from build123d import *

# Parameters (mm, degrees)
SKETCH2_R          = 4.7625
SKETCH3_R          = 1.7272
CUT_EXTRUDE1_DEPTH = 12.7


with BuildPart() as part:
    # Base-Sweep: sweep along a path in Sketch1
    with BuildLine(Plane(origin=(0, 0, 0), x_dir=(0, 0, -1), z_dir=(1, 0, 0))) as base_sweep_path:
        Line((0, 0), (0, 21.59))
        ThreePointArc((0, 21.59), (1.859871939, 26.080128061), (6.35, 27.94))
        Line((6.35, 27.94), (82.55, 27.94))
        ThreePointArc((82.55, 27.94), (87.040128061, 26.080128061), (88.9, 21.59))
        Line((88.9, 21.59), (88.9, 0))
    # Sketch2 → Base-Sweep (sweep)
    with BuildSketch(Plane(origin=(0, 0, 0), x_dir=(1, 0, 0), z_dir=(0, 1, 0))):
        Circle(SKETCH2_R)
    sweep(path=base_sweep_path.line)

    # Sketch3 → Cut-Extrude1 (cut)
    with BuildSketch(Plane.XZ):
        Circle(SKETCH3_R)
        with Locations((0, -88.9)):
            Circle(SKETCH3_R)
    extrude(amount=-CUT_EXTRUDE1_DEPTH, mode=Mode.SUBTRACT)


solid = part.part
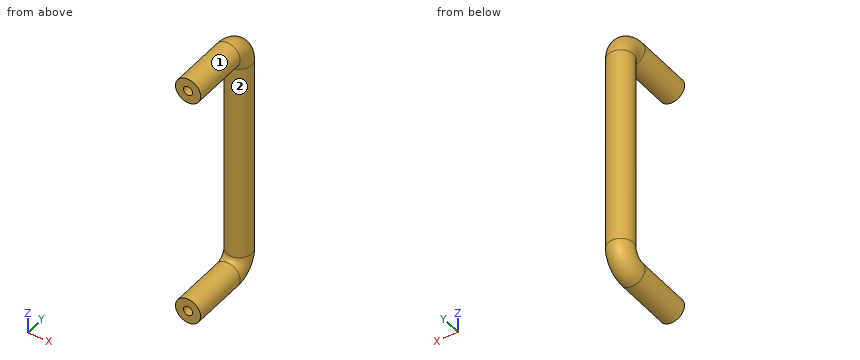
CAD build for the part. Positions are in the model's coordinates, mm. Face numbers are marked on the shaded views. A direction names the side the tool comes from. Coordinates: 2 decimals unless noted, no trailing zeros. Order: outer loops, then holes, each group sorted by start corner. A loop starts at its lowest first (then second) coordinate and runs counter-clockwise, first axis right, second up.
Item 1: Pin check, flat tips, straight feed: pin 1 Ø2 at (x, z) = (-2.5, -41.5) entering from -Y; pin 2 Ø1.7 at (x, z) = (0.5, -0.5) entering from -Y; pin 3 Ø8 at (y, z) = (26, -50) entering from -X; pin 4 Ø2 at (x, z) = (0, -88.9) entering from +Y. Stop position of each tip, or through.
Check sheet entries:
pin 1: stops at y = 23.42
pin 2: stops at y = 12.7
pin 3: stops at x = -4.76
pin 4: stops at y = 31.33
Item 2: Band-saw the part on C-C on z = -69.5. List the corners of the cut face in (x, y) (1 decimal).
Check sheet entries:
outline: circle Ø9.5 at (0, 27.9)
Item 3: Drill centre lines: L1, parallel to Z at x = 0, y = 9; L2, parallel to Z at x = -1, y = 7; L3, parallel to Z at x = 0, y = 23. Where is each one in solid material? Low to high.
Check sheet entries:
L1: z = -93.66 to -90.63, -87.17 to -84.14, -4.76 to -1.73, 1.73 to 4.76
L2: z = -93.56 to -90.31, -87.49 to -84.24, -4.66 to -1.41, 1.41 to 4.66
L3: z = -93.57 to -83.28, -5.62 to 4.67
Item 4: Band-saw the part on A-A on y = 11. List the corners of the cut face in (x, z) (1 decimal).
Check sheet entries:
outline: circle Ø9.5 at (0, -88.9); circle Ø9.5 at (0, 0); hole circle Ø3.5 at (0, -88.9); hole circle Ø3.5 at (0, 0)
Item 5: 3-axis set-ups, long thin cutter, end or side, ignore diameter. For the marked faces 1 and 2: which of +Z, -Z, +X, -X, +Y, -Y reach the whole face in a straight line?
Check sheet entries:
face 1: -Y
face 2: none
